Can you work these out from the model? Positions are in its coordinate system, mm. Give positions to 0.01 mm unless a question says otherwise; leave off trailing zeros. Order: outer loops, then holes, each group sorted by start corner. A loop starts at its lowest first (then second) coordinate and runs counter-clockwise, first axis right, second up. Notation, with made-up numbers: (80.25, -32) -> (94.25, -32) arc R7 cw to (94.25, -24) -> close; hole circle Ø8 at (89, 68). An arc over 180 degrees is marked (long way). Answer as CSV lines item,"result".
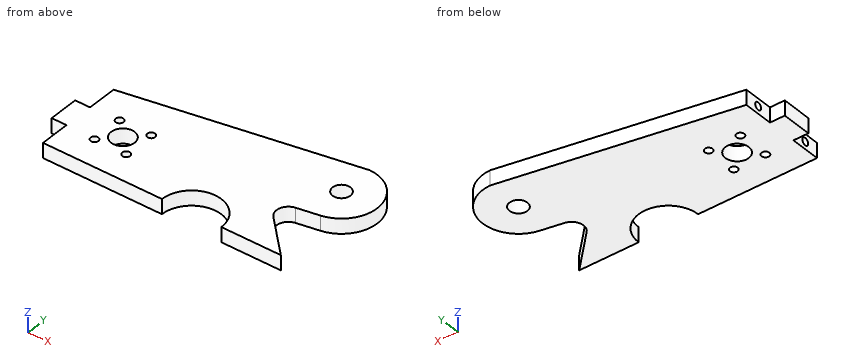
```python
from build123d import *

# Parameters (mm, degrees)
SKETCH1_R           = 3.81
SKETCH1_R_2         = 1.651
BOSS_EXTRUDE1_DEPTH = 6.35
FILLET2_R           = 5.08
SKETCH3_R           = 1.5875
CUT_EXTRUDE1_DEPTH  = 6.35
CUT_EXTRUDE2_DEPTH  = 6.35
SKETCH7_R           = 5.000000033
CUT_EXTRUDE3_DEPTH  = 125.084268237


with BuildPart() as part:
    # Sketch1 → Boss-Extrude1 (new body)
    with BuildSketch(Plane.XY):
        with BuildLine():
            Line((0, 0), (101.6, 0))
            Line((101.6, 0), (79.43330905, 22.16669095))
            Line((79.43330905, 22.16669095), (98.16062093, 25.658150496))
            ThreePointArc((98.16062093, 25.658150496), (110.542778436, 42.04253584), (95.367453293, 55.88))
            Line((95.367453293, 55.88), (0, 38.1))
            Line((0, 38.1), (0, 25.4))
            Line((0, 25.4), (-6.35, 25.4))
            Line((-6.35, 25.4), (-6.35, 12.7))
            Line((-6.35, 12.7), (0, 12.7))
            Line((0, 12.7), (0, 0))
        make_face()
        with Locations((95.367453293, 40.64)):
            Circle(SKETCH1_R, mode=Mode.SUBTRACT)
        with Locations((25.817011896, 25.817011896)):
            Circle(SKETCH1_R_2, mode=Mode.SUBTRACT)
        with Locations((25.817011896, 12.282988104)):
            Circle(SKETCH1_R_2, mode=Mode.SUBTRACT)
        with Locations((12.282988104, 12.282988104)):
            Circle(SKETCH1_R_2, mode=Mode.SUBTRACT)
        with Locations((12.282988104, 25.817011896)):
            Circle(SKETCH1_R_2, mode=Mode.SUBTRACT)
    extrude(amount=BOSS_EXTRUDE1_DEPTH)

    # Fillet2
    fillet2_edges = [part.edges().sort_by_distance(p)[0] for p in [
        (79.43330905, 22.16669095, 3.175),
    ]]
    fillet(fillet2_edges, radius=FILLET2_R)

    # Sketch3 → Cut-Extrude1 (cut)
    with BuildSketch(Plane.ZY):
        with Locations(Location((3.175, 31.75, 0), (0, 0, 270))):
            Circle(SKETCH3_R)
        with Locations(Location((3.175, 6.35, 0), (0, 0, 270))):
            Circle(SKETCH3_R)
    extrude(amount=-CUT_EXTRUDE1_DEPTH, mode=Mode.SUBTRACT)

    # Sketch6 → Cut-Extrude2 (cut)
    with BuildSketch(Plane.XY.offset(6.35)):
        with BuildLine():
            Line((50.8, 0), (76.2, 0))
            ThreePointArc((76.2, 0), (63.5, 12.7), (50.8, 0))
        make_face()
    extrude(amount=-CUT_EXTRUDE2_DEPTH, mode=Mode.SUBTRACT)

    # Sketch7 → Cut-Extrude3 (cut, through all)
    with BuildSketch(Plane.XY.offset(6.35)):
        with Locations((19.05, 19.05)):
            Circle(SKETCH7_R)
    extrude(amount=-CUT_EXTRUDE3_DEPTH, mode=Mode.SUBTRACT)


solid = part.part
```
Item 1: Please list where these lines run through material, in increasing order: line 1 along Z through (x, y) = (2, 31.75); line 2 along X through (y, z) = (11.5, 0.75); line 3 along X through (y, z) = (20, 4.5).
Numbers:
line 1,"z = 0 to 1.59, 4.76 to 6.35"
line 2,"x = 0 to 10.83, 13.74 to 24.36, 27.27 to 58.11, 68.89 to 90.1"
line 3,"x = -6.35 to 14.14, 23.96 to 84.88"
Item 2: Imagine slicing it at C-C, the plane y = 6.35. Please give me the cut outline in (x, z), then the cut area to 3 significant figures.
Numbers:
outline,"(0, 0) -> (52.5, 0) -> (52.5, 6.35) -> (0, 6.35) -> (0, 4.76) -> (6.35, 4.76) -> (6.35, 1.59) -> (0, 1.59) -> close; (74.5, 0) -> (95.25, 0) -> (95.25, 6.35) -> (74.5, 6.35) -> close"
area,"445 mm²"
Item 3: For pin 1 (3 mm diameter, centred on x = 61.5, z = 5, fed in from -Y); pin 2 (3 mm diameter, centred on y = 30.5, z = 2, fed in from -X); pin 3 (1.6 mm diameter, centred on y = 6.5, z = 3, fed in from -X), each with a flat end and sliding along its axis, tell me the tip position at first contact or that it passes through.
Numbers:
pin 1,"stops at y = 12.21"
pin 2,"stops at x = 0"
pin 3,"stops at x = 6.35"
Item 4: Imagine slicing it at B-B, the plane x = 19.05. Please give me the cut outline in (y, z).
Numbers:
outline,"(0, 0) -> (14.05, 0) -> (14.05, 6.35) -> (0, 6.35) -> close; (24.05, 0) -> (41.65, 0) -> (41.65, 6.35) -> (24.05, 6.35) -> close"
Item 5: Imagine slicing it at A-A, the plane y = 40.64. Please give me the cut outline in (x, z), then the cut area to 3 significant figures.
Numbers:
outline,"(13.62, 0) -> (91.56, 0) -> (91.56, 6.35) -> (13.62, 6.35) -> close; (99.18, 0) -> (110.61, 0) -> (110.61, 6.35) -> (99.18, 6.35) -> close"
area,"567 mm²"
Item 6: Imagine slicing it at D-D, the plane x = 75. Please give me the cut outline in (y, z), then the cut area to 3 significant figures.
Numbers:
outline,"(5.39, 0) -> (52.08, 0) -> (52.08, 6.35) -> (5.39, 6.35) -> close"
area,"297 mm²"
